Autodesk Inventor part; units mm, degrees
ref_plane "YZ Plane" through (0, 0, 0) normal (1, 0, 0) x (0, 1, 0)
ref_plane "XZ Plane" through (0, 0, 0) normal (0, 1, 0) x (-1, 0, 0)
ref_plane "XY Plane" through (0, 0, 0) normal (0, 0, 1) x (1, 0, 0)
sketch "Sketch1" plane through (0, 0, 0) normal (0, 1, 0) x (-1, 0, 0)
  circle A0 centre (0, 0) radius 41.5 construction
  line L0 (0, -41.5) -> (0, 41.5)
  arc A1 (0, 41.5) -> (0, -41.5) centre (0, 0) ccw
  circle A2 centre (-6, -34) radius 2.5
  circle A3 centre (-6, 34) radius 2.5
  line L1 (0, 0) -> (-41.5, 0) construction
  circle A4 centre (-35, 0) radius 2.5
  circle A5 centre (0, 0) radius 35.5 construction
  line L2 (0, 0) -> (-20.75, -35.9401) construction
  line L3 (0, 0) -> (-38.9972, -14.1938) construction
  arc A6 (-33.3591, -12.1417) -> (-17.75, -30.7439) centre (0, 0) ccw construction
  arc A7 (-35.7083, -12.9968) -> (-19, -32.909) centre (0, 0) ccw
  arc A8 (-31.0099, -11.2867) -> (-16.5, -28.5788) centre (0, 0) ccw
  arc A9 (-31.0099, -11.2867) -> (-35.7083, -12.9968) centre (-33.3591, -12.1417) ccw
  arc A10 (-19, -32.909) -> (-16.5, -28.5788) centre (-17.75, -30.7439) ccw
  arc A11 (-19, 32.909) -> (-35.7083, 12.9968) centre (0, 0) ccw
  arc A12 (-16.5, 28.5788) -> (-31.0099, 11.2867) centre (0, 0) ccw
  arc A13 (-35.7083, 12.9968) -> (-31.0099, 11.2867) centre (-33.3591, 12.1417) ccw
  arc A14 (-16.5, 28.5788) -> (-19, 32.909) centre (-17.75, 30.7439) ccw
  dimension "d2" = 83
  dimension "d3" = 83
  dimension "d4" = 5
  dimension "d5" = 6
  dimension "d6" = 34
  dimension "d7" = 34
  dimension "d8" = 35
  dimension "d11" = 6
  dimension "d12" = 20
  dimension "d13" = 30
  dimension "d14" = 5
extrude "Extrusion1" add sketch "Sketch1" along normal blind 2
sketch "Dimen. Arduino" plane through (0, 2, 0) normal (0, 1, 0) x (1, 0, 0)
  line L0 (0, 0) -> (41.5, 0) construction
  arc A0 (0, -41.5) -> (0, 41.5) centre (0, 0) ccw construction
  line L1 (3.11, -21.59) -> (20.89, -21.59) construction
  line L2 (20.89, -21.59) -> (20.89, 21.59) construction
  line L3 (20.89, 21.59) -> (3.11, 21.59) construction
  line L4 (3.11, 21.59) -> (3.11, -21.59) construction
  line L5 (3.11, -21.59) -> (20.89, 21.59) construction
  line L6 (20.89, -21.59) -> (3.11, 21.59) construction
  line L7 (19.62, -20.32) -> (4.38, -20.32) construction
  line L8 (4.38, -20.32) -> (4.38, 20.32) construction
  line L9 (4.38, 20.32) -> (19.62, 20.32) construction
  line L10 (19.62, 20.32) -> (19.62, -20.32) construction
  line L11 (19.62, -20.32) -> (4.38, 20.32) construction
  line L12 (4.38, -20.32) -> (19.62, 20.32) construction
  circle A1 centre (4.38, 20.32) radius 0.75
  circle A2 centre (19.62, 20.32) radius 0.75
  circle A3 centre (4.38, -20.32) radius 0.75
  circle A4 centre (19.62, -20.32) radius 0.75
  point P0 (12, 0)
  dimension "d17" = 43.18
  dimension "d18" = 17.78
  dimension "d19" = 12
  dimension "d20" = 1.27
  dimension "d21" = 1.27
  dimension "d22" = 1.5
extrude "Extrusion2" cut sketch "Dimen. Arduino" against normal through all
fillet "Fillet1" radius 1 16 edges at (25.2795, 2, 21.212) (34.2141, 2, 9.7925) (29.1097, 2, 24.4259) (15.5849, 2, 31.9939) (15.5849, 2, -31.9939) (29.1097, 2, -24.4259) (34.2141, 2, -9.7925) (25.2795, 2, -21.212) (29.1097, 0, 24.4259) (15.5849, 0, 31.9939) (25.2795, 0, 21.212) (34.2141, 0, 9.7925) (25.2795, 0, -21.212) (15.5849, 0, -31.9939) (29.1097, 0, -24.4259) (34.2141, 0, -9.7925)
properties part number "_3DPrint"
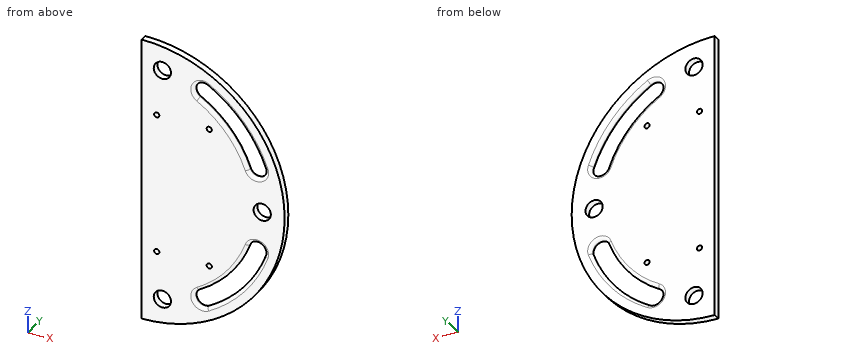
Work out the finished part from the listing and answer in its coordinate system (mm). Give positions to 0.01 mm unless a question says otherwise; leave off trailing zeros. Write each loop counter-clockwise with the first axis right and the second up, starting at its lowest first coordinate (ties: lowest second). Pieces come first, ordered by that corner, then holes. Notation, with made-up numbers: (28.25, 62.5) - (84.25, 62.5) arc R20 ccw to (84.25, 73.5) - close; hole circle Ø7 at (56, 21.25). An arc over 180 degrees is marked (long way). One line per item, written item: value. Start each with the question number.
1. Given pin 1 (1 mm diameter, centred on x = 23.5, z = -31.5, fed in from -Y); pin 2 (1 mm diameter, centred on x = 8.5, y = 1.5, fed in from -Z); pin 3 (1.5 mm diameter, centred on x = 16.5, z = -33, fed in from +Y), each flat-ended and moving along its own axis, determine where each tip first touches the part or whether it passes through.
2. Find section C-C (x = 4.38). Write down the section's boundary in (y, z), then the cut area to 3 significant figures.
3. Find section A-A (z = 0). Write down the section's boundary in (x, y), then the cut area to 3 significant figures.
4. Consider probe 1 along Z at (x, y) = (19.62, 1.5); probe 2 along Z at (x, y) = (18.5, 0.3); probe 3 along Z at (x, y) = (25.5, 0.3). Determine where each line is inside the solid, lowest interval first.
5. Find section B-B (y = 0.5). State how many separate pieces and enclosed holes the cut face has, then the cut area to 3 significant figures.
Geometry results:
1. pin 1: y = 0
1. pin 2: z = -40.72
1. pin 3: y = 1.99
2. outline: (0, -41.27) - (2, -41.27) - (2, -35.9) - (0, -35.9) - close; (0, -32.1) - (2, -32.1) - (2, -21.07) - (0, -21.07) - close; (0, -19.57) - (2, -19.57) - (2, 19.57) - (0, 19.57) - close; (0, 21.07) - (2, 21.07) - (2, 32.1) - (0, 32.1) - close; (0, 35.9) - (2, 35.9) - (2, 41.27) - (0, 41.27) - close
2. area: 144 mm2
3. outline: (0, 0) - (32.5, 0) - (32.5, 2) - (0, 2) - close; (37.5, 0) - (41.5, 0) - (41.5, 2) - (37.5, 2) - close
3. area: 73.0 mm2
4. probe 1: -36.57 to -32.7, -26.37 to -21.07, -19.57 to 19.57, 21.07 to 26.37, 32.7 to 36.57
4. probe 2: -37.15 to -33.43, -26.98 to 26.98, 33.43 to 37.15
4. probe 3: -32.74 to -28.56, -20.49 to 20.49, 28.56 to 32.74
5. separate pieces: 1
5. enclosed holes: 9
5. area: 2,330 mm2
